from build123d import *

# Parameters (mm, degrees)
SKETCH1_W           = 40
SKETCH1_H           = 20
BOSS_EXTRUDE1_DEPTH = 40
CUT_EXTRUDE1_DEPTH  = 20


with BuildPart() as part:
    # Sketch1 → Boss-Extrude1 (new body)
    with BuildSketch(Plane.XY):
        Polygon((20, -30), (-20, -30), (0, 0), (40, 0), align=None)
        with Locations((20, 10)):
            Rectangle(SKETCH1_W, SKETCH1_H)
    extrude(amount=BOSS_EXTRUDE1_DEPTH)

    # Sketch2 → Cut-Extrude1 (cut)
    with BuildSketch(Plane(origin=(0, 20, 0), x_dir=(1, 0, 0), z_dir=(0, 1, 0))):
        Polygon((0, -40), (40, 0), (40, -40), align=None)
    extrude(amount=-CUT_EXTRUDE1_DEPTH, mode=Mode.SUBTRACT)


solid = part.part
Can you work these out from the model? Positions are in its coordinate system, mm. A direction names the side the tool comes from. Round coordinates to 2 decimals unless told otherwise and drop trailing zeros. Loops run counter-clockwise (first coordinate to the right, second up) from the corner with the lowest first, then second, coordinate; pieces in that order, holes last. Notation, with made-up numbers: (0, 75.25) - (22, 75.25) arc R17 cw to (22, 84.25) - close; hole circle Ø7 at (84, 45). An arc over 180 degrees is marked (long way). Use CSV: the item, a comma, the result in double quotes. Start each with the question number.
1) If we section it at A-A on z = 12: Write out the boundary of the cut face in (x, y).
2) Please list where these lines run through material, in increasing order: probe 1 along Z at (x, y) = (20, 16); probe 2 along Y at (x, z) = (9.5, 33); probe 3 along Y at (x, z) = (-7, 25). Write a range as [from, to].
3) If we section it at B-B on x = 34.5: Write out the boundary of the cut face in (y, z).
4) If we section it at D-D on y = 8: Write out the boundary of the cut face in (x, z).
5) If we section it at C-C on z = 24: Write out the boundary of the cut face in (x, y), plus the area to 3 significant figures.
6) For faces 1 (the flat face through (15, 20, 15)), 2 (the flat face through (0, 10, 20)), 3 (the flat face through (20, 10, 20)), which set-ups out of +Z, -Z, +X, -X, +Y, -Y let a thin tool reach every point of the face, with its end or its side?
7) For pin 1 Ø3 at (y, z) = (-17, 9.5) entering from -X; pin 2 Ø12 at (x, y) = (23.5, 11.5) entering from +Z; pin 3 Ø16 at (y, z) = (9, 16.5) entering from -X, each with a flat end and sliding along its axis, tell me the tip position at first contact or that it passes through.
Geometry results:
1,outline,"(-20, -30) - (20, -30) - (40, 0) - (28, 0) - (28, 20) - (0, 20) - (0, 0) - close"
2,probe 1,"z = [0, 20]"
2,probe 2,"y = [-30, 0]"
2,probe 3,"y = [-30, -10.5]"
3,outline,"(-8.25, 0) - (20, 0) - (20, 5.5) - (0, 5.5) - (0, 40) - (-8.25, 40) - close"
4,outline,"(0, 0) - (40, 0) - (0, 40) - close"
5,outline,"(-20, -30) - (20, -30) - (40, 0) - (16, 0) - (16, 20) - (0, 20) - (0, 0) - close"
5,area,"1,520 mm2"
6,face 1,"+Z, -Z, +X, -X, +Y"
6,face 2,"+Z, -Z, -X, +Y"
6,face 3,"+Z, +X, +Y"
7,pin 1,"stops at x = -12.33"
7,pin 2,"stops at z = 22.5"
7,pin 3,"stops at x = 0"
